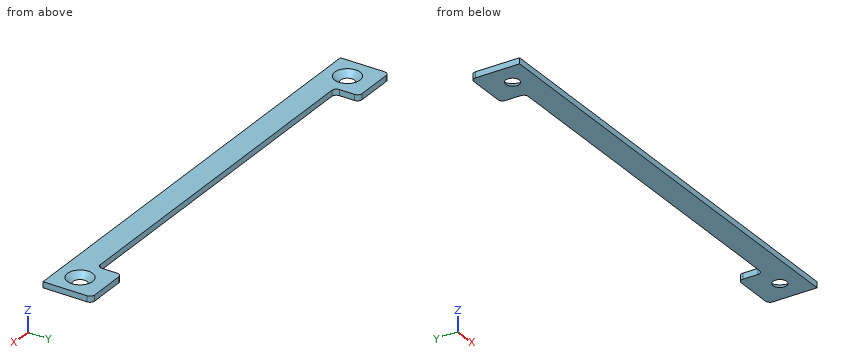
```python
from build123d import *

# Parameters (mm, degrees)
BOSS_EXTRUDE1_DEPTH                          = 1.27
FILLET1_R                                    = 1
CSK_FOR_M2_5_COUNTERSUNK_RAISED_HEAD_2_COUNT = 2
CSK_FOR_M2_5_COUNTERSUNK_RAISED_HEAD_2_PITCH = 89.03694267


with BuildPart() as part:
    # Sketch1 → Boss-Extrude1 (new body)
    with BuildSketch(Plane.XY):
        Polygon((-38.499957014, 0), (60.560042986, 0), (60.560042986, 10.550876612), (50.560042986, 10.550876612), (50.560042986, 5.275438306), (-28.499957014, 5.275438306), (-28.499957014, 10.550876612), (-38.499957014, 10.550876612), align=None)
    extrude(amount=BOSS_EXTRUDE1_DEPTH)

    # Fillet1
    fillet1_edges = [part.edges().sort_by_distance(p)[0] for p in [
        (-38.499957014, 10.550876612, 0.635),
        (-28.499957014, 10.550876612, 0.635),
        (-28.499957014, 5.275438306, 0.635),
        (50.560042986, 5.275438306, 0.635),
        (50.560042986, 10.550876612, 0.635),
        (60.560042986, 10.550876612, 0.635),
    ]]
    fillet(fillet1_edges, radius=FILLET1_R)

    # Sketch6 → CSK for M2.5 Countersunk Raised Head Screw1 (revolve, cut)
    with BuildSketch(Plane(origin=(-33.476617277, 4.775438306, 1.27), x_dir=(0, -1, 0), z_dir=(1, 0, 0))):
        Polygon((0, 0), (0, 1.27), (1.45, 1.27), (1.45, 1.3), (2.75, 0), align=None)
    csk_for_m2_5_countersunk_raised_head_scr = revolve(axis=Axis((-33.476617277, 4.775438306, 7.62), (0, 0, -1)), mode=Mode.SUBTRACT)

    # CSK for M2.5 Countersunk Raised Head 2: CSK for M2.5 Countersunk Raised Head Screw1 ×2
    with Locations(*[(i * CSK_FOR_M2_5_COUNTERSUNK_RAISED_HEAD_2_PITCH, 0, 0) for i in range(1, CSK_FOR_M2_5_COUNTERSUNK_RAISED_HEAD_2_COUNT)]):
        add(csk_for_m2_5_countersunk_raised_head_scr, mode=Mode.SUBTRACT)


solid = part.part
```
The listing builds one solid part. Answer for the finished solid, in the listing's coordinates (mm). Round coordinates to 2 decimals unless told otherwise and drop trailing zeros. Loops run counter-clockwise (first coordinate to the right, second up) from the corner with the lowest first, then second, coordinate; pieces in that order, holes last.
Q1. Section B-B, the plane x = 43 is taken. Determine the outline of the cut face in (y, z), then the cut area to 3 significant figures.
Q2. Find the intervals of material crossed by line 1 (X direction, y = 9, z = 0.4); line 2 (X direction, y = 5.5, z = 0.95); line 3 (X direction, y = 3.5, z = 0.65), in increasing order.
Q3. Given pin 1 Ø0.6 at (x, z) = (9, 0.5) entering from +Y, flat-ended and moving along its own axis, determine where the tip first touches the part or whether it passes through.
Q4. Section A-A, the plane z = 0.6 is taken. Determine the outline of the cut face in (x, y), then the cut area to 3 significant figures.
Completed:
1. outline: (0, 0) - (5.28, 0) - (5.28, 1.27) - (0, 1.27) - close
1. area: 6.70 mm2
2. line 1: x = -38.5 to -28.5, 50.56 to 60.56
2. line 2: x = -38.5 to -35.8, -31.16 to -28.13, 50.19 to 53.24, 57.88 to 60.56
2. line 3: x = -38.5 to -35.18, -31.77 to 53.85, 57.27 to 60.56
3. pin 1: stops at y = 5.28
4. outline: (-38.5, 0) - (60.56, 0) - (60.56, 9.55) arc R1 ccw to (59.56, 10.55) - (51.56, 10.55) arc R1 ccw to (50.56, 9.55) - (50.56, 6.28) arc R1 cw to (49.56, 5.28) - (-27.5, 5.28) arc R1 cw to (-28.5, 6.28) - (-28.5, 9.55) arc R1 ccw to (-29.5, 10.55) - (-37.5, 10.55) arc R1 ccw to (-38.5, 9.55) - close; hole circle Ø4.16 at (-33.48, 4.78); hole circle Ø4.16 at (55.56, 4.78)
4. area: 600 mm2
